```python
from build123d import *

# Parameters (mm, degrees)
F1_W     = 30
F1_H     = 35
F2_DEPTH = 1
F3_W     = 6.3
F3_H     = 6.75
F4_DEPTH = 2
F5_R     = 1.3
F6_DEPTH = 3.001
F7_W     = 17.4
F7_H     = 21.5
F8_DEPTH = 1.001


with BuildPart() as f2:
    # F1 (on Top) → F2 (new body)
    with BuildSketch(Plane.XY):
        with Locations((11.7, 13.75)):
            Rectangle(F1_W, F1_H)
    extrude(amount=F2_DEPTH)

    # F3 (on face) → F4 (join)
    with BuildSketch(Plane.XY.offset(1)):
        with Locations((-0.15, 27.875)):
            Rectangle(F3_W, F3_H)
        with Locations((23.55, 27.875)):
            Rectangle(F3_W, F3_H)
        with Locations((23.55, -0.375)):
            Rectangle(F3_W, F3_H)
        with Locations((-0.15, -0.375)):
            Rectangle(F3_W, F3_H)
    extrude(amount=F4_DEPTH)

    # F5 (on face) → F6 (cut, through all)
    with BuildSketch(Plane.XY.offset(3)):
        with Locations((0, 27.5)):
            Circle(F5_R)
        with Locations((23.4, 27.5)):
            Circle(F5_R)
        with Locations((23.4, 0)):
            Circle(F5_R)
        Circle(F5_R)
    extrude(amount=-F6_DEPTH, mode=Mode.SUBTRACT)

    # F7 (on face) → F8 (cut, through all)
    with BuildSketch(Plane.XY.offset(1)):
        with Locations((11.7, 13.75)):
            Rectangle(F7_W, F7_H)
    extrude(amount=-F8_DEPTH, mode=Mode.SUBTRACT)


solid = f2.part
```
Model file for the job. Use its own axes, mm. A direction names the side the tool comes from. Give positions to 0.01 mm unless a question says otherwise; leave off trailing zeros. Write each loop counter-clockwise with the first axis right and the second up, starting at its lowest first coordinate (ties: lowest second). Pieces come first, ordered by that corner, then holes. Notation, with made-up numbers: (-18.5, 69.5) - (36.5, 69.5) arc R23 cw to (36.5, 106.5) - close; hole circle Ø6 at (84.25, 74.25). An arc over 180 degrees is marked (long way). One line per question, with ' | ' between items. Start each with the question number.
(1) Slice it at B-B on x = 19. Write the cut outline in (y, z), plus the area to 3 significant figures.
(2) 3-axis set-ups, long thin cutter, end or side, ignore diameter. For faces 1 (the face through (3, 0, 2)), 2 (the face through (0, 14, 1)), 3 (the face through (11.6, 3, 0.5)): which of +Z, -Z, +X, -X, +Y, -Y reach the whole face in a straight line?
(3) Slice it at C-C on y = 27.5. Write the cut outline in (x, z).
(4) Slice it at A-A on z = 1.95. Write the cut outline in (x, y).
(5) Pin check, flat tips, straight feed: P1, Ø5, axis at x = 12, y = 2.5, coming from the -Z side; P2, Ø3.5, axis at x = 12, y = 29.5, coming from the +Z side; P3, Ø1.6, axis at x = 0, y = 0, coming from the -Z side. Stop position of each tip, or through.
(6) Wall check: line 1 along Y through (x, z) = (23.4, 1.6); line 2 along Y through (x, z) = (23.4, 0.7); line 3 along X through (y, z) = (23, 0.3). Give the ranges that are in metal, low to high. Write a range as from..to.
(7) Slice it at D-D on x = 0. Write the cut outline in (y, z).
(8) Two-plate mould, pull along Y, no slides. Class faces 4 (the face through (24, 3, 2)), 5 (the face through (20.4, 28, 2)), 6 (the face through (24.6, 27, 1.5)): +Y half, -Y half, draft (parallel to the pull), parting line (faces both ways), or undercut.
Results below:
1) outline: (-3.75, 0) - (3, 0) - (3, 1) - (-3.75, 1) - close; (24.5, 0) - (31.25, 0) - (31.25, 1) - (24.5, 1) - close | area: 13.5 mm^2
2) face 1: +Z, +Y, -Y | face 2: +Z, +X, -X | face 3: +Z, -Z
3) outline: (-3.3, 0) - (-1.3, 0) - (-1.3, 3) - (-3.3, 3) - close; (1.3, 0) - (22.1, 0) - (22.1, 3) - (20.4, 3) - (20.4, 1) - (3, 1) - (3, 3) - (1.3, 3) - close; (24.7, 0) - (26.7, 0) - (26.7, 3) - (24.7, 3) - close
4) outline: (-3.3, -3.75) - (3, -3.75) - (3, 3) - (-3.3, 3) - close; (-3.3, 24.5) - (3, 24.5) - (3, 31.25) - (-3.3, 31.25) - close; (20.4, -3.75) - (26.7, -3.75) - (26.7, 3) - (20.4, 3) - close; (20.4, 24.5) - (26.7, 24.5) - (26.7, 31.25) - (20.4, 31.25) - close; hole circle Ø2.6 at (0, 0); hole circle Ø2.6 at (0, 27.5); hole circle Ø2.6 at (23.4, 0); hole circle Ø2.6 at (23.4, 27.5)
5) P1: z = 0 | P2: z = 1 | P3: through
6) line 1: -3.75..-1.3, 1.3..3, 24.5..26.2, 28.8..31.25 | line 2: -3.75..-1.3, 1.3..26.2, 28.8..31.25 | line 3: -3.3..3, 20.4..26.7
7) outline: (-3.75, 0) - (-1.3, 0) - (-1.3, 3) - (-3.75, 3) - close; (1.3, 0) - (26.2, 0) - (26.2, 3) - (24.5, 3) - (24.5, 1) - (3, 1) - (3, 3) - (1.3, 3) - close; (28.8, 0) - (31.25, 0) - (31.25, 3) - (28.8, 3) - close
8) face 4: undercut | face 5: draft | face 6: undercut
